Solid Edge part; units mm, degrees
sketch "Sketch1" plane through (0, 0, 0) normal (0, 0, 1) x (1, 0, 0)
  line L0 (-30.4449, 6) -> (347.1507, 6)
  arc A0 (347.1507, 6) -> (351.3257, 4.904) centre (347.1507, -2.5) cw
  line L1 (351.3257, 4.904) -> (373.3271, -7.5022)
  arc A1 (373.3271, -7.5022) -> (368.3271, -19.6127) centre (370.0853, -13.2512) cw
  line L2 (368.3271, -19.6127) -> (321.7315, -6.7349)
  line L3 (-12.1244, -6.5) -> (320, -6.5)
  line L4 (-28.1811, -10.693) -> (-13.8555, -6.7348)
  arc A2 (-28.1811, -10.693) -> (-30.4449, 6) centre (-30.4449, -2.5) cw
  arc A3 (320, -6.5) -> (321.7315, -6.7349) centre (320, -13) cw
  arc A4 (-13.8555, -6.7348) -> (-12.1244, -6.5) centre (-12.1244, -13) cw
  line L5 (347.1507, 4) -> (-30.4449, 4)
  line L6 (-28.7137, -8.7652) -> (-14.3881, -4.807)
  line L7 (320, -4.5) -> (-12.1244, -4.5)
  line L8 (368.8599, -17.6849) -> (322.2643, -4.8071)
  line L9 (350.3433, 3.1619) -> (372.3447, -9.2443)
  arc A5 (-28.7137, -8.7652) -> (-30.4449, 4) centre (-30.4449, -2.5) cw
  arc A6 (-14.3881, -4.807) -> (-12.1244, -4.5) centre (-12.1244, -13) cw
  arc A7 (320, -4.5) -> (322.2643, -4.8071) centre (320, -13) cw
  arc A8 (368.8599, -17.685) -> (372.3447, -9.2443) centre (370.0853, -13.2512) ccw
  arc A9 (347.1507, 4) -> (350.3433, 3.1619) centre (347.1507, -2.5) cw
extrude "Protrusion1" add sketch "Sketch1" along normal blind 6
properties material "PVC"
Here's how the part is built. I have some questions about the finished solid (model axes, mm). A direction names the side the tool comes from. Coordinates: 2 decimals unless noted, no trailing zeros. Loops run counter-clockwise (first coordinate to the right, second up) from the corner with the lowest first, then second, coordinate; pieces in that order, holes last. Notation, with made-up numbers: (-17.5, 47.5) - (7.5, 47.5) arc R11 ccw to (7.5, 52.5) - close; hole circle Ø7 at (53.5, 48.25). An arc over 180 degrees is marked (long way). Return JSON: item names as keys, results as strings. Group by question number.
Item 1: We'd pull the mould along X, two halves only. Please class faces 1 (the face through (345.888, -11.336, 2.958)), 2 (the face through (362.17, -1.21, 2.96)), 3 (the face through (170, -5, 0)), 4 (the face through (361.19, -2.954, 2.958)): +X half, -X half, draft (parallel to the pull), parting line (faces both ways), or undercut.
Item 2: On a 3-axis mill with a long thin cutter (end or side, diameter ignored), from which of +Z, -Z, +X, -X, +Y, -Y can I reach the whole of each face in a straight line? I mean faces 5 (the face through (170, -5, 6)), 6 (the face through (345.355, -13.264, 2.958)). Say none if no direction works.
Item 3: Will these pins go through, and if not, where does the flat tip stop? P1, Ø2, axis at y = -8.5, z = 2.5, coming from the +X side; P2, Ø2, axis at y = -6, z = 3.5, coming from the -X side; P3, Ø8, axis at x = -30.44, y = -2.5, coming from the -Z side.
Item 4: If we section it at C-C on y = -0.25: Write out the boundary of the cut face in (x, z).
Item 5: If we section it at B-B on z = 2.9: Write out the boundary of the cut face in (x, y), and give its area (3 significant figures).
Item 6: If we section it at A-A on x = 265: Write out the boundary of the cut face in (y, z), and give its area (3 significant figures).
Item 7: I need wall thicknesses on line 1 (Y direction, x = 35, z = 0.7); line 2 (X direction, y = -2.5, z = 3.6). Which ranges of each line are inside material? Lowest first, please. Write a range as from..to.
Calculated:
{
 "1": {"face 1": "undercut", "face 2": "+X half", "face 3": "draft", "face 4": "undercut"},
 "2": {"face 5": "+Z, +X, -X, +Y, -Y", "face 6": "+Z, -Z, -Y"},
 "3": {"P1": "stops at x = 375.52", "P2": "stops at x = -38.57", "P3": "passes through"},
 "4": {"outline": "(-38.64, 0) - (-36.54, 0) - (-36.54, 6) - (-38.64, 6) - close; (356.39, 0) - (360.47, 0) - (360.47, 6) - (356.39, 6) - close"},
 "5": {"outline": "(-30.44, 6) arc R8.5 ccw (long way) to (-28.18, -10.69) - (-13.86, -6.73) arc R6.5 cw to (-12.12, -6.5) - (320, -6.5) arc R6.5 cw to (321.73, -6.73) - (368.33, -19.61) arc R6.6 ccw to (373.33, -7.5) - (351.33, 4.9) arc R8.5 ccw to (347.15, 6) - close; hole (-30.44, 4) arc R6.5 ccw (long way) to (-28.71, -8.77) - (-14.39, -4.81) arc R8.5 cw to (-12.12, -4.5) - (320, -4.5) arc R8.5 cw to (322.26, -4.81) - (368.86, -17.68) arc R4.6 ccw to (372.34, -9.24) - (350.34, 3.16) arc R6.5 ccw to (347.15, 4) - close", "area": "1,700 mm^2"},
 "6": {"outline": "(-6.5, 0) - (-4.5, 0) - (-4.5, 6) - (-6.5, 6) - close; (4, 0) - (6, 0) - (6, 6) - (4, 6) - close", "area": "24.0 mm^2"},
 "7": {"line 1": "y = -6.5..-4.5, 4..6", "line 2": "x = -38.94..-36.94, 360.38..364.46"}
}
